Autodesk Inventor part; units mm, degrees
ref_plane "YZ Plane" through (0, 0, 0) normal (1, 0, 0) x (0, 1, 0)
ref_plane "XZ Plane" through (0, 0, 0) normal (0, 1, 0) x (-1, 0, 0)
ref_plane "XY Plane" through (0, 0, 0) normal (0, 0, 1) x (1, 0, 0)
sketch "Sketch1" plane through (0, 0, 0) normal (0, 0, 1) x (1, 0, 0)
  line L0 (-21.5, 51.7145) -> (21.5, 51.7145)
  line L1 (21.5, 51.7145) -> (21.5, -51.7145)
  line L2 (-21.5, -51.7145) -> (-21.5, 51.7145)
  line L3 (5.5, -51.7145) -> (5.5, -48.7145)
  line L4 (1.5, -46.7145) -> (2.65, -46.7145)
  line L5 (2.65, -46.7145) -> (2.65, -44.3145)
  line L6 (2.65, -44.3145) -> (1.5, -44.3145)
  line L7 (1.5, -44.3145) -> (1.5, -43.7145)
  line L8 (1.5, -43.7145) -> (-1.5, -43.7145)
  line L9 (-1.5, -43.7145) -> (-1.5, -44.3145)
  line L10 (-1.5, -44.3145) -> (-2.65, -44.3145)
  line L11 (-2.65, -44.3145) -> (-2.65, -46.7145)
  line L12 (-2.65, -46.7145) -> (-1.5, -46.7145)
  line L13 (-5.5, -48.7145) -> (-5.5, -51.7145)
  line L14 (1.5, -46.7145) -> (1.5, -48.7145)
  line L15 (1.5, -48.7145) -> (5.5, -48.7145)
  line L16 (-1.5, -46.7145) -> (-1.5, -48.7145)
  line L17 (-1.5, -48.7145) -> (-5.5, -48.7145)
  line L18 (21.5, -51.7145) -> (13.5, -51.7145)
  line L19 (-5.5, -51.7145) -> (-21.5, -51.7145)
  line L20 (-30.1, 0) -> (30.1, 0) construction
  line L21 (0, -72.4008) -> (0, 72.4004) construction
  line L22 (13.5, 44.7145) -> (13.5, 51.7145)
  line L23 (13.5, 51.7145) -> (10.5, 51.7145)
  line L24 (10.5, 44.7145) -> (10.5, 51.7145)
  line L25 (13.5, 44.7145) -> (10.5, 44.7145)
  line L26 (13.5, -4.1443) -> (13.5, 18.7145)
  line L27 (13.5, 18.7145) -> (10.5, 18.7145)
  line L28 (10.5, -4.1443) -> (10.5, 18.7145)
  line L29 (13.5, -4.1443) -> (10.5, -4.1443)
  line L30 (13.5, -51.7149) -> (13.5, -30.1443)
  line L31 (13.5, -30.1443) -> (10.5, -30.1443)
  line L32 (10.5, -51.7149) -> (10.5, -30.1443)
  line L33 (13.5, -51.7149) -> (10.5, -51.7149)
  line L34 (16.5, 41.7145) -> (16.5, 34.3645)
  line L35 (16.5, 41.7145) -> (13.5, 41.7145)
  line L36 (13.5, 34.3645) -> (13.5, 41.7145)
  line L37 (16.5, 34.3645) -> (13.5, 34.3645)
  line L38 (16.5, 29.0645) -> (16.5, 21.7145)
  line L39 (16.5, 29.0645) -> (13.5, 29.0645)
  line L40 (13.5, 21.7145) -> (13.5, 29.0645)
  line L41 (16.5, 21.7145) -> (13.5, 21.7145)
  line L42 (16.5, -7.1443) -> (16.5, -14.4943)
  line L43 (16.5, -7.1443) -> (13.5, -7.1443)
  line L44 (13.5, -14.4943) -> (13.5, -7.1443)
  line L45 (16.5, -14.4943) -> (13.5, -14.4943)
  line L46 (16.5, -19.7943) -> (16.5, -27.1443)
  line L47 (16.5, -19.7943) -> (13.5, -19.7943)
  line L48 (13.5, -27.1443) -> (13.5, -19.7943)
  line L49 (16.5, -27.1443) -> (13.5, -27.1443)
  line L50 (-13.5, -19.7943) -> (-13.5, -27.1443)
  line L51 (-13.5, -19.7943) -> (-16.5, -19.7943)
  line L52 (-16.5, -27.1443) -> (-16.5, -19.7943)
  line L53 (-13.5, -27.1443) -> (-16.5, -27.1443)
  line L54 (-13.5, -7.1443) -> (-13.5, -14.4943)
  line L55 (-13.5, -7.1443) -> (-16.5, -7.1443)
  line L56 (-16.5, -14.4943) -> (-16.5, -7.1443)
  line L57 (-13.5, -14.4943) -> (-16.5, -14.4943)
  line L58 (-13.5, 29.0645) -> (-13.5, 21.7145)
  line L59 (-13.5, 29.0645) -> (-16.5, 29.0645)
  line L60 (-16.5, 21.7145) -> (-16.5, 29.0645)
  line L61 (-13.5, 21.7145) -> (-16.5, 21.7145)
  line L62 (-13.5, 41.7145) -> (-13.5, 34.3645)
  line L63 (-13.5, 41.7145) -> (-16.5, 41.7145)
  line L64 (-16.5, 34.3645) -> (-16.5, 41.7145)
  line L65 (-13.5, 34.3645) -> (-16.5, 34.3645)
  line L66 (16.5, 34.3645) -> (13.5, 29.0645) construction
  line L67 (13.5, 34.3645) -> (16.5, 29.0645) construction
  line L68 (13.5, -14.4943) -> (16.5, -19.7943) construction
  line L69 (16.5, -14.4943) -> (13.5, -19.7943) construction
  line L70 (-13.5, -14.4943) -> (-16.5, -19.7943) construction
  line L71 (-16.5, -14.4943) -> (-13.5, -19.7943) construction
  line L72 (-13.5, 34.3645) -> (-16.5, 29.0645) construction
  line L73 (-16.5, 34.3645) -> (-13.5, 29.0645) construction
  circle A0 centre (-15, 31.7145) radius 1.4
  circle A1 centre (15, 31.7145) radius 1.4
  circle A2 centre (15, -17.1443) radius 1.4
  circle A3 centre (-15, -17.1443) radius 1.4
  line L74 (13.5, -51.7145) -> (10.5, -51.7145)
  line L75 (10.5, -51.7145) -> (5.5, -51.7145)
  dimension "d0" = 43
  dimension "d12" = 3
  dimension "d13" = 5.3
  dimension "d15" = 2.4
  dimension "d19" = 3
  dimension "d20" = 5
  dimension "d21" = 8
  dimension "d25" = 103.429
  dimension "d26" = 2.8
  dimension "d27" = 2.8
  dimension "d28" = 2.8
  dimension "d29" = 2.8
  dimension "d30" = 5
extrude "Extrusion1" add sketch "Sketch1" along normal blind 3 contours L0 L24 L25 L22 L1 L18 L30 L31 L32 L75 L3 L15 L14 L4 L5 L6 L7 L8 L9 L10 L11 L12 L16 L17 L13 L19 L2
properties part number "Y-Shafts-Holder_Side"
Part model, mm, in its own coordinate system. A direction names the side the tool comes from. Round coordinates to 2 decimals unless told otherwise and drop trailing zeros. Write each loop counter-clockwise with the first axis right and the second up, starting at its lowest first coordinate (ties: lowest second). Pieces come first, ordered by that corner, then holes. Notation, with made-up numbers: (82.5, -12) -> (108.5, -12) arc R18 cw to (108.5, 14) -> close; hole circle Ø1 at (36, 37). An arc over 180 degrees is marked (long way). Return JSON: item names as keys, results as strings. Group by question number.
Q1. Which spindle directions (+Z, -Z, +X, -X, +Y, -Y) get a long thin tool onto all of the face, cutting with end or side? Do faces 1 (the flat face through (17, 51.714, 1)), 2 (the flat face through (12, -30.144, 1)), 3 (the flat face through (13.5, 48, 1)), 4 (the flat face through (-15, -27.144, 1)). Say none if no direction does.
Q2. Pin check, flat tips, straight feed: pin 1 (2.5 mm diameter, centred on x = 15, y = 31.71, fed in from +Z); pin 2 (0.9 mm diameter, centred on x = -0.5, z = 2, fed in from -Y). Stop position of each tip, or through.
Q3. Mould opens along X. For faces 5 (the flat face through (18, -51.714, 1)), 6 (the flat face through (15, 29.064, 1)), 7 (the flat face through (13.5, 38, 1)) say: pulls with the +X half, pulls with the -X half, needs draft (parallel to the pull), parting line crosses it, or undercut.
Q4. Saw through at D-D on x = 0.5. Write the cut outline in (y, z), plus the area to 3 significant figures.
Q5. Saw through at A-A on x = 15. Write the cut outline in (y, z).
Q6. Saw through at C-C on y = 27. Write the cut outline in (x, z), plus the area to 3 significant figures.
Q7. Probe L1, parallel to X at y = -22, z = 2.7; L2, parallel to X at y = -37, z = 1.7; L3, parallel to X at y = -16.5, z = 1.85. List the from-to ranges inside material, lowest first. Write a range as [from, to].
Q8. Saw through at B-B on y = 12.5. Write the cut outline in (x, z), plus the area to 3 significant figures.
Answer:
{
 "1": {"face 1": "+Z, -Z, +X, -X, +Y", "face 2": "+Z, -Z, -Y", "face 3": "+Z, -Z, +Y", "face 4": "+Z, -Z"},
 "2": {"pin 1": "through", "pin 2": "y = -43.71"},
 "3": {"face 5": "needs draft", "face 6": "undercut", "face 7": "undercut"},
 "4": {"outline": "(-43.71, 0) -> (51.71, 0) -> (51.71, 3) -> (-43.71, 3) -> close", "area": "286 mm2"},
 "5": {"outline": "(-51.71, 0) -> (-27.14, 0) -> (-27.14, 3) -> (-51.71, 3) -> close; (-19.79, 0) -> (-18.54, 0) -> (-18.54, 3) -> (-19.79, 3) -> close; (-15.74, 0) -> (-14.49, 0) -> (-14.49, 3) -> (-15.74, 3) -> close; (-7.14, 0) -> (21.71, 0) -> (21.71, 3) -> (-7.14, 3) -> close; (29.06, 0) -> (30.31, 0) -> (30.31, 3) -> (29.06, 3) -> close; (33.11, 0) -> (34.36, 0) -> (34.36, 3) -> (33.11, 3) -> close; (41.71, 0) -> (51.71, 0) -> (51.71, 3) -> (41.71, 3) -> close"},
 "6": {"outline": "(-21.5, 0) -> (-16.5, 0) -> (-16.5, 3) -> (-21.5, 3) -> close; (-13.5, 0) -> (13.5, 0) -> (13.5, 3) -> (-13.5, 3) -> close; (16.5, 0) -> (21.5, 0) -> (21.5, 3) -> (16.5, 3) -> close", "area": "111 mm2"},
 "7": {"L1": "[-21.5, -16.5], [-13.5, 13.5], [16.5, 21.5]", "L2": "[-21.5, 10.5], [13.5, 21.5]", "L3": "[-21.5, -16.24], [-13.76, 13.76], [16.24, 21.5]"},
 "8": {"outline": "(-21.5, 0) -> (10.5, 0) -> (10.5, 3) -> (-21.5, 3) -> close; (13.5, 0) -> (21.5, 0) -> (21.5, 3) -> (13.5, 3) -> close", "area": "120 mm2"}
}
